from build123d import *

# Parameters (mm, degrees)
PAD_DEPTH       = 30
SKETCH001_R     = 2.65
POCKET_DEPTH    = 5
SKETCH002_R     = 2.65
SKETCH002_R_2   = 1.5
POCKET001_DEPTH = 5


with BuildPart() as part:
    # Sketch → Pad (new body)
    with BuildSketch(Plane.XY):
        Polygon((-45, -10), (-30, -10), (-30, 5), (30, 5), (30, -10), (45, -10), (45, -5), (35, -5), (35, 10), (-35, 10), (-35, -5), (-45, -5), align=None)
    extrude(amount=PAD_DEPTH)

    # Sketch001 (on Face11 of Pad) → Pocket (cut)
    with BuildSketch(Plane(origin=(0, -5, 0), x_dir=(-1, 0, 0), z_dir=(0, 1, 0))):
        with Locations((-40, 25)):
            Circle(SKETCH001_R)
        with Locations((-40, 5)):
            Circle(SKETCH001_R)
        with Locations((40, 25)):
            Circle(SKETCH001_R)
        with Locations((40, 5)):
            Circle(SKETCH001_R)
    extrude(amount=-POCKET_DEPTH, mode=Mode.SUBTRACT)

    # Sketch002 (on Face15 of Pocket) → Pocket001 (cut)
    with BuildSketch(Plane(origin=(0, 10, 0), x_dir=(-1, 0, 0), z_dir=(0, 1, 0))):
        with Locations((0, 15)):
            Circle(SKETCH002_R)
        with Locations((-15, 20)):
            Circle(SKETCH002_R_2)
        with Locations((-15, 10)):
            Circle(SKETCH002_R_2)
        with Locations((15, 20)):
            Circle(SKETCH002_R_2)
        with Locations((15, 10)):
            Circle(SKETCH002_R_2)
    extrude(amount=-POCKET001_DEPTH, mode=Mode.SUBTRACT)


solid = part.part
Model file for the job. Use its own axes, mm. A direction names the side the tool comes from. Round coordinates to 2 decimals unless told otherwise and drop trailing zeros. Order: outer loops, then holes, each group sorted by start corner. A loop starts at its lowest first (then second) coordinate and runs counter-clockwise, first axis right, second up.
(1) Pin check, flat tips, straight feed: pin 1 (5 mm diameter, centred on x = 15, z = 10, fed in from -Y); pin 2 (7.5 mm diameter, centred on y = 5.5, z = 8, fed in from -X); pin 3 (12 mm diameter, centred on y = 6, z = 8, fed in from +X). Stop position of each tip, or through.
(2) Band-saw the part on D-D (y = 3.5). List the corners of the cut face in (x, z).
(3) Band-saw the part on A-A (y = -6.25). List the corners of the cut face in (x, z), then the cut area to 3 significant figures.
(4) Band-saw the part on C-C (z = 15). List the corners of the cut face in (x, y), then the cut area to 4 significant figures.
(5) 3-axis set-ups, long thin cutter, end or side, ignore diameter. For faces 4 (the face through (40, -5, 15)), 5 (the face through (-38, -10, 15)), 6 (the face through (0, 10, 11)), 7 (the face through (-40, -5, 15)), 8 (the face through (0, 5, 11)): which of +Z, -Z, +X, -X, +Y, -Y reach the whole face in a straight line?
(6) Drill centre lines: line 1 (Z direction, x = 40, y = -6.05); line 2 (Z direction, x = 15, y = 8.1); line 3 (Z direction, x = 0, y = 6.5). Where is each one in solid material? Low to high.
(7) Band-saw the part on B-B (x = 40). List the corners of the cut face in (y, z), then the cut area to 3 significant figures.
(8) Pull direction X, two halves, no side cores. Call faces 1 (the face through (-35, 3, 15)), 2 (the face through (-4, 6, 0)), 3 (the face through (-13.5, 7.54, 10.07)): released by +X, released by -X, zero draft, split by the parting line, or undercut.
Verdict:
1. pin 1: stops at y = 5
1. pin 2: stops at x = -35
1. pin 3: stops at x = 35
2. outline: (-35, 0) - (-30, 0) - (-30, 30) - (-35, 30) - close; (30, 0) - (35, 0) - (35, 30) - (30, 30) - close
3. outline: (-45, 0) - (-30, 0) - (-30, 30) - (-45, 30) - close; (30, 0) - (45, 0) - (45, 30) - (30, 30) - close; hole circle Ø5.3 at (-40, 5); hole circle Ø5.3 at (-40, 25); hole circle Ø5.3 at (40, 5); hole circle Ø5.3 at (40, 25)
3. area: 812 mm2
4. outline: (-45, -10) - (-30, -10) - (-30, 5) - (-2.65, 5) - (-2.65, 10) - (-35, 10) - (-35, -5) - (-45, -5) - close; (2.65, 5) - (30, 5) - (30, -10) - (45, -10) - (45, -5) - (35, -5) - (35, 10) - (2.65, 10) - close
4. area: 573.5 mm2
5. face 4: +Z, -Z, +X, +Y
5. face 5: +Z, -Z, +X, -X, -Y
5. face 6: +Z, -Z, +X, -X, +Y
5. face 7: +Z, -Z, -X, +Y
5. face 8: +Z, -Z, -Y
6. line 1: z = 0 to 2.35, 7.65 to 22.35, 27.65 to 30
6. line 2: z = 0 to 8.5, 11.5 to 18.5, 21.5 to 30
6. line 3: z = 0 to 12.35, 17.65 to 30
7. outline: (-10, 0) - (-5, 0) - (-5, 2.35) - (-10, 2.35) - close; (-10, 7.65) - (-5, 7.65) - (-5, 22.35) - (-10, 22.35) - close; (-10, 27.65) - (-5, 27.65) - (-5, 30) - (-10, 30) - close
7. area: 97.0 mm2
8. face 1: released by -X
8. face 2: zero draft
8. face 3: undercut
